Here's how the part is built. I have some questions about the finished solid (model axes, mm). A direction names the side the tool comes from. Coordinates: 2 decimals unless noted, no trailing zeros. Order: outer loops, then holes, each group sorted by start corner. A loop starts at its lowest first (then second) coordinate and runs counter-clockwise, first axis right, second up. Notation, with made-up numbers: (80.25, 80.25) - (114.25, 80.25) arc R15 cw to (114.25, 92.25) - close; hole circle Ø6 at (-18, 39.25). An arc over 180 degrees is marked (long way). Use one line per item in the form item = value. Start each with the question number.
from build123d import *

# Parameters (mm, degrees)
SKETCH1_R           = 55
BOSS_EXTRUDE1_DEPTH = 5
SKETCH2_R           = 11.5
SKETCH2_R_2         = 10
BOSS_EXTRUDE2_DEPTH = 10
SKETCH3_R           = 10
CUT_EXTRUDE1_DEPTH  = 79.421935707


with BuildPart() as part:
    # Sketch1 → Boss-Extrude1 (new body)
    with BuildSketch(Plane.XY):
        Circle(SKETCH1_R)
    extrude(amount=BOSS_EXTRUDE1_DEPTH)

    # Sketch2 → Boss-Extrude2 (add)
    with BuildSketch(Plane.XY.offset(5)):
        Circle(SKETCH2_R)
        Circle(SKETCH2_R_2, mode=Mode.SUBTRACT)
    extrude(amount=BOSS_EXTRUDE2_DEPTH)

    # Sketch3 → Cut-Extrude1 (cut, through all)
    with BuildSketch(Plane.XY.offset(5)):
        Circle(SKETCH3_R)
    extrude(amount=-CUT_EXTRUDE1_DEPTH, mode=Mode.SUBTRACT)


solid = part.part
1) Suppose I cut it at C-C, the plane z = 11.5. List the corners of the cut face in (x, y) for me, then the cut area to 3 significant figures.
2) I need wall thicknesses on probe 1 along Y at (x, z) = (0, 11.5); probe 2 along Y at (x, z) = (0, 3.95); probe 3 along Z at (x, y) = (-15, 23). Which ranges of each line are inside material? Lowest first, please. Write a range as [from, to].
3) For pin 1 (8 mm diameter, centred on x = 8.5, y = 34, fed in from +Z); pin 2 (1 mm diameter, centred on x = -7, z = 9, fed in from -Y); pin 3 (1.5 mm diameter, centred on y = -8, z = 3.5, fed in from -X), each with a flat end and sliding along its axis, tell me the tip position at first contact or that it passes through.
4) Suppose I cut it at A-A, the plane y = 0. List the corners of the cut face in (x, z) for me.
5) Which directions (+Z, -Z, +X, -X, +Y, -Y) give clear straight access to the entire face, cutting with the end or side of a thin tool? Please do faces 1 (the flat face through (-1, -11, 0)), 2 (the cylindrical face through (-1.5, 11.4, 9.9)).
6) Suppose I cut it at D-D, the plane z = 3.5. List the corners of the cut face in (x, y) for me, then the cut area to 3 significant figures.
From the geometry:
q1.outline = circle Ø23 at (0, 0); hole circle Ø20 at (0, 0)
q1.area = 101 mm2
q2.probe_1 = [-11.5, -10], [10, 11.5]
q2.probe_2 = [-55, -10], [10, 55]
q2.probe_3 = [0, 5]
q3.pin_1 = 5
q3.pin_2 = -9.49
q3.pin_3 = -54.52
q4.outline = (-55, 0) - (-10, 0) - (-10, 15) - (-11.5, 15) - (-11.5, 5) - (-55, 5) - close; (10, 0) - (55, 0) - (55, 5) - (11.5, 5) - (11.5, 15) - (10, 15) - close
q5.face_1 = -Z, +X, -X, +Y, -Y
q5.face_2 = +Z
q6.outline = circle Ø110 at (0, 0); hole circle Ø20 at (0, 0)
q6.area = 9,190 mm2
